```python
from build123d import *

# Parameters (mm, degrees)
SKETCH1_W           = 15
SKETCH1_H           = 50
BOSS_EXTRUDE1_DEPTH = 10
SKETCH2_W           = 0.85
SKETCH2_H           = 1.5
CUT_EXTRUDE1_DEPTH  = 52.53882032
CUT_EXTRUDE3_DEPTH  = 54.150729064


with BuildPart() as part:
    # Sketch1 → Boss-Extrude1 (new body)
    with BuildSketch(Plane(origin=(0, 0, 0), x_dir=(0, 0, -1), z_dir=(1, 0, 0))):
        with Locations((0, 25)):
            Rectangle(SKETCH1_W, SKETCH1_H)
    extrude(amount=BOSS_EXTRUDE1_DEPTH)

    # Sketch2 → Cut-Extrude1 (cut, through all)
    with BuildSketch(Plane(origin=(10, 0, 0), x_dir=(0, 0, -1), z_dir=(1, 0, 0))):
        with Locations((-7.075, 5)):
            Rectangle(SKETCH2_W, SKETCH2_H)
        with Locations((7.075, 5)):
            Rectangle(SKETCH2_W, SKETCH2_H)
    extrude(amount=-CUT_EXTRUDE1_DEPTH, mode=Mode.SUBTRACT)

    # Sketch3 → Cut-Extrude3 (cut, through all)
    with BuildSketch(Plane.XY.offset(7.5)):
        Polygon((2.90122494, 50), (10, 8.648873186), (10, 50), align=None)
    extrude(amount=-CUT_EXTRUDE3_DEPTH, mode=Mode.SUBTRACT)


solid = part.part
```
The model under review builds one solid part; all positions refer to its coordinate system, in mm. A direction names the side the tool comes from. Give positions to 0.01 mm unless a question says otherwise; leave off trailing zeros. Write each loop counter-clockwise with the first axis right and the second up, starting at its lowest first coordinate (ties: lowest second). Pieces come first, ordered by that corner, then holes. Notation, with made-up numbers: M -1,33.5 L 31,33.5 A21 cw 31,44.5 Z; hole C -40,16.5 d2. An arc over 180 degrees is marked long. Write item = value, one per line. Start each with the question number.
Q1. For line 1 (X direction, y = 20, z = -5); line 2 (X direction, y = 19, z = -4.75), list the stretches that pass through material, from the lowest coordinate up.
Q2. We need section A-A (z = -5.75). State the section outline as (x, y) points.
Q3. We need section D-D (x = 8.5). State the section outline as (y, z) points, plus the area to 3 significant figures.
Q4. Mouldability with a two-part tool opening along Y and no side actions: class faces 1 (the face through (10, 4, 0)), 2 (the face through (5, 5.75, 7)), 3 (the face through (5, 0, 0)) as released by +Y, released by -Y, zero draft, split by the parting line, or undercut.
Q5. We need section B-B (x = 4.25). State the section outline as (y, z) points.
Q6. We need section C-C (y = 40.5). State the section outline as (x, z) points, plus the area to 3 significant figures.
Q7. Machinability: for faces 4 (the face through (5, 2, 7.5)), 5 (the face through (5, 4.25, 7)), 6 (the face through (5, 5, -6.65)), which of the approach directions +Z, -Z, +X, -X, +Y, -Y give a long, thin tool a straight path to every point of the face, cutting with its end or side? Answer none if there is none.
Q8. Clearance check with flat-ended pins moving along their axes: pin 1 (0.9 mm diameter, centred on x = 6, z = 7, fed in from -Y); pin 2 (3 mm diameter, centred on y = 20.5, z = -2, fed in from +X); pin 3 (1.2 mm diameter, centred on x = 7, y = 5, fed in from +Z); pin 4 (0.8 mm diameter, centred on x = 6, y = 5, fed in from -Z). State where each tip first meets the part, or that it passes through.
Result set:
q1.line_1 = 0 to 8.05
q1.line_2 = 0 to 8.22
q2.outline = M 0,0 L 10,0 L 10,8.65 L 2.9,50 L 0,50 Z
q3.outline = M 0,-7.5 L 4.25,-7.5 L 4.25,-6.65 L 5.75,-6.65 L 5.75,-7.5 L 17.39,-7.5 L 17.39,7.5 L 5.75,7.5 L 5.75,6.65 L 4.25,6.65 L 4.25,7.5 L 0,7.5 Z
q3.area = 258 mm2
q4.face_1 = zero draft
q4.face_2 = undercut
q4.face_3 = released by -Y
q5.outline = M 0,-7.5 L 4.25,-7.5 L 4.25,-6.65 L 5.75,-6.65 L 5.75,-7.5 L 42.14,-7.5 L 42.14,7.5 L 5.75,7.5 L 5.75,6.65 L 4.25,6.65 L 4.25,7.5 L 0,7.5 Z
q6.outline = M 0,-7.5 L 4.53,-7.5 L 4.53,7.5 L 0,7.5 Z
q6.area = 68.0 mm2
q7.face_4 = +Z, +X, -X, +Y, -Y
q7.face_5 = +Z, +X, -X
q7.face_6 = -Z, +X, -X
q8.pin_1 = 0
q8.pin_2 = 8.22
q8.pin_3 = 6.65
q8.pin_4 = -6.65
